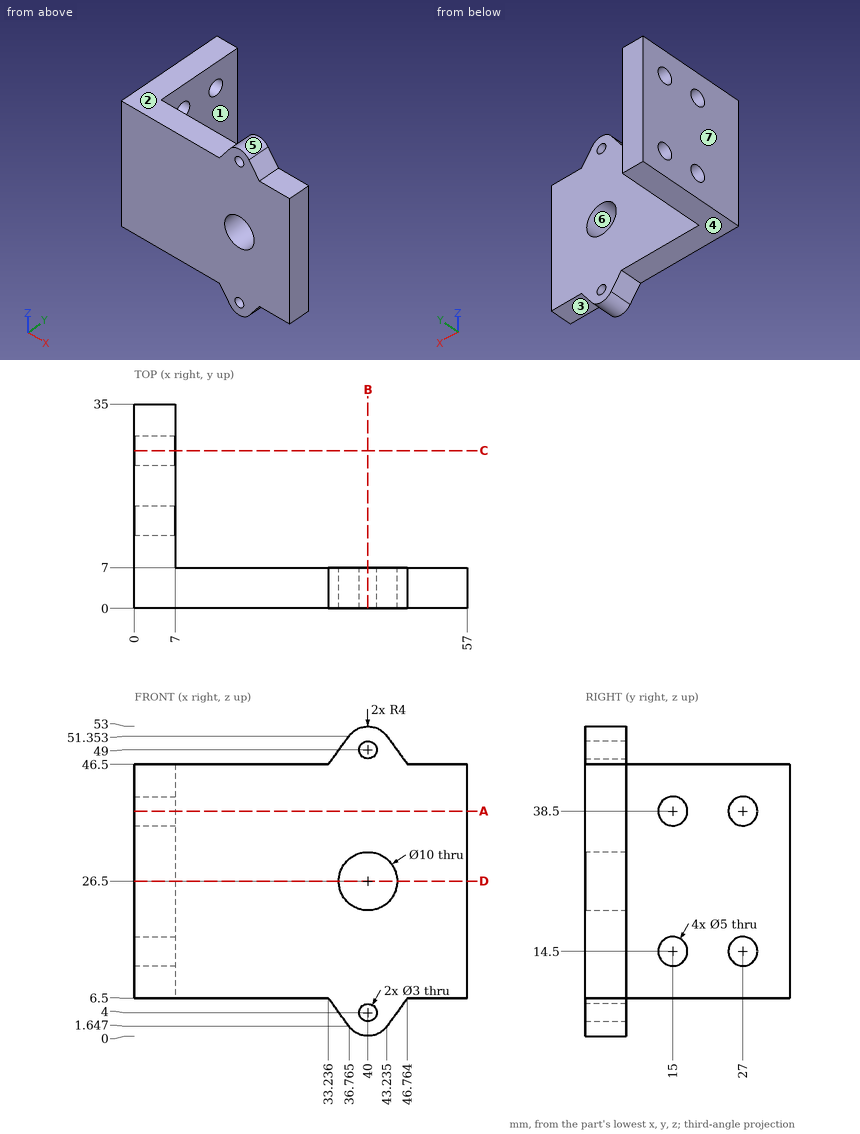
Verification items for this drawing (mm, ordinates from the low corner). A direction names the side the tool comes from. Coordinates: 2 decimals unless noted, no trailing zeros. Loops run counter-clockwise (first coordinate to the right, second up) from the corner with the lowest first, then second, coordinate; pieces in that order, holes last. Notation, with made-up numbers: (81, 82) - (93, 82) arc R13 ccw to (93, 88) - close; hole circle Ø7 at (7.25, 28). An arc over 180 degrees is marked (long way). Answer as a JSON object with one key per item and string values.
(1) Scan lines: line 1 along Z through (x, y) = (3, 27); line 2 along Y through (x, z) = (8, 32.5). Record each from-to range of solid material in increasing order.
Response:
{"line 1": "z = 6.5 to 12, 17 to 36, 41 to 46.5", "line 2": "y = 0 to 7"}
(2) Cross-section at A-A, the plane z = 38.5. Record the boundary of the cut face in (x, y), then the cut area to 3 significant figures.
Response:
{"outline": "(0, 0) - (57, 0) - (57, 7) - (7, 7) - (7, 12.5) - (0, 12.5) - close; (0, 17.5) - (7, 17.5) - (7, 24.5) - (0, 24.5) - close; (0, 29.5) - (7, 29.5) - (7, 35) - (0, 35) - close", "area": "525 mm²"}
(3) Mould release check, pull along Z, two halves, no side actions. Record for the marked faces 5, 6 and 7: pulls with the +Z half, pulls with the -Z half, needs draft (parallel to the pull), parting line crosses it, or undercut.
Response:
{"face 5": "pulls with the +Z half", "face 6": "undercut", "face 7": "needs draft"}
(4) Go/stop test with flat-tipped pins: pin 1 Ø8 at (y, z) = (15, 14.5) entering from +X; pin 2 Ø25 at (x, z) = (40.5, 36.5) entering from +Y; pin 3 Ø2 at (x, y) = (51, 2.5) entering from +Z; pin 4 Ø2.5 at (x, z) = (40, 49) entering from +Y. Record where each tip stops, or that it passes through.
Response:
{"pin 1": "stops at x = 7", "pin 2": "stops at y = 7", "pin 3": "stops at z = 46.5", "pin 4": "passes through"}
(5) Cross-section at B-B, the plane x = 40. Record the boundary of the cut face in (y, z).
Response:
{"outline": "(0, 0) - (7, 0) - (7, 2.5) - (0, 2.5) - close; (0, 5.5) - (7, 5.5) - (7, 21.5) - (0, 21.5) - close; (0, 31.5) - (7, 31.5) - (7, 47.5) - (0, 47.5) - close; (0, 50.5) - (7, 50.5) - (7, 53) - (0, 53) - close"}
(6) Cross-section at D-D, the plane z = 26.5. Record the boundary of the cut face in (x, y).
Response:
{"outline": "(0, 0) - (35, 0) - (35, 7) - (7, 7) - (7, 35) - (0, 35) - close; (45, 0) - (57, 0) - (57, 7) - (45, 7) - close"}
(7) Cross-section at C-C, the plane y = 27. Record the boundary of the cut face in (x, z).
Response:
{"outline": "(0, 6.5) - (7, 6.5) - (7, 12) - (0, 12) - close; (0, 17) - (7, 17) - (7, 36) - (0, 36) - close; (0, 41) - (7, 41) - (7, 46.5) - (0, 46.5) - close"}
(8) Access from +Z, -Z, +X, -X, +Y, -Y to the whole of each face (thin tool, end or side, straight path). Record for the marked faces 1, 2, 3 and 4.
Response:
{"face 1": "+Z, -Z, +X, +Y", "face 2": "+Z, -X, +Y, -Y", "face 3": "-Z, +X, +Y, -Y", "face 4": "-Z, -X, +Y, -Y"}
